from build123d import *

# Parameters (mm, degrees)
F0_W     = 250
F0_H     = 75
F1_DEPTH = 17.5
F3_DEPTH = 35.001
F4_R     = 9.5
F5_DEPTH = 50
F6_W     = 15
F6_H     = 150
F7_DEPTH = 37.501


with BuildPart() as f1:
    # F0 (on Right) → F1 (new body, symmetric)
    with BuildSketch(Plane.YZ):
        Rectangle(F0_W, F0_H)
    extrude(amount=F1_DEPTH, both=True)

    # F2 (on face) → F3 (cut, through all)
    with BuildSketch(Plane(origin=(-17.5, 0, 0), x_dir=(0, -1, 0), z_dir=(-1, 0, 0))):
        with BuildLine():
            ThreePointArc((-125, 37.5), (-59.748084, 27.923052), (0, 0))
            ThreePointArc((0, 0), (61.011045, -23.713184), (125, -37.5))
            Line((125, -37.5), (125, 37.5))
            Line((125, 37.5), (-125, 37.5))
        make_face()
        with BuildLine():
            Line((-125, -37.5), (76.611606, -37.5))
            ThreePointArc((76.611606, -37.5), (52.114015, -27.662953), (26.677744, -20.59927))
            ThreePointArc((26.677744, -20.59927), (-50.552427, -16.563242), (-125, -37.5))
        make_face()
        with BuildLine():
            ThreePointArc((26.677744, -20.59927), (-49.327107, -2.636934), (-125, -21.950044))
            Line((-125, -21.950044), (-125, -37.5))
            ThreePointArc((-125, -37.5), (-50.552427, -16.563242), (26.677744, -20.59927))
        make_face()
    extrude(amount=-F3_DEPTH, mode=Mode.SUBTRACT)

    # F4 (on face) → F5 (cut)
    with BuildSketch(Plane(origin=(0, 125, 0), x_dir=(-1, 0, 0), z_dir=(0, 1, 0))):
        with Locations((0, 17.31561)):
            Circle(F4_R)
    extrude(amount=-F5_DEPTH, mode=Mode.SUBTRACT)

    # F6 (on Top) → F7 (cut, through all)
    with BuildSketch(Plane.XY):
        with Locations((0.914634, -15.109161)):
            Rectangle(F6_W, F6_H)
    extrude(amount=-F7_DEPTH, mode=Mode.SUBTRACT)


solid = f1.part
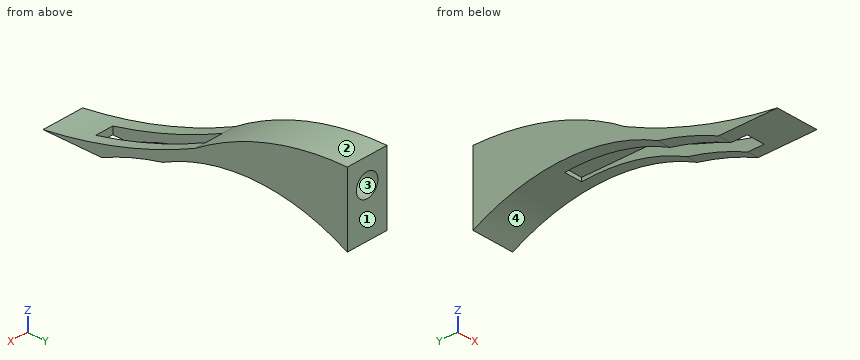
Read the model definition and answer for the solid it produces. Units are mm, in the model's axes. Face numbers are marked on the shaded views. Give positions to 0.01 mm unless a question says otherwise; leave off trailing zeros. Write each loop counter-clockwise with the first axis right and the second up, starting at its lowest first coordinate (ties: lowest second). Pieces come first, ordered by that corner, then holes. Notation, with made-up numbers: (-32, 41.5) -> (27, 41.5) arc R28 cw to (27, 61.5) -> close; hole circle Ø5 at (-10.75, 87.5). An arc over 180 degrees is marked (long way). Answer as a JSON object with one key per item and string values. Group by question number.
1) Find section B-B (z = -12.5). Write down the section's boundary in (x, y).
2) Find section D-D (y = -65). Write down the section's boundary in (x, z).
3) Find section A-A (x = 0). Write down the section's boundary in (y, z), and give its area (3 significant figures).
4) Each of these flat-tipped pins is pushed along its axis until it touches: P1, Ø1.9, axis at x = 0, z = -33.5, coming from the +Y side; P2, Ø1.5, axis at x = -4.5, y = -90, coming from the +Z side; P3, Ø10, axis at x = 9.5, y = -22, coming from the +Z side. Where does it stop, or does it pass through?
5) Consider L1, parallel to X at y = -56, z = -25; L2, parallel to Z at x = 0, y = 87.5; L3, parallel to Z at x = 0, y = 101. Determine where each line is inside the solid, lowest interval first. Write a range as from..to.
6) The mould has two halves that part along Y. Classify the marked faces 1, 2, 3 and 4: +Y half, -Y half, draft (parallel to the pull), parting line (faces both ways), or undercut.
7) Find section C-C (x = 14). Write down the section's boundary in (y, z), and give its area (3 significant figures).
Values follow:
{
 "1": {"outline": "(-17.5, -28.59) -> (-6.59, -28.59) -> (-6.59, -8.1) -> (-17.5, -8.1) -> close; (-17.5, 103.84) -> (17.5, 103.84) -> (17.5, 125) -> (-17.5, 125) -> close; (8.41, -28.59) -> (17.5, -28.59) -> (17.5, -8.1) -> (8.41, -8.1) -> close"},
 "2": {"outline": "(-17.5, -32.44) -> (-6.59, -32.44) -> (-6.59, -24.89) -> (-17.5, -24.89) -> close; (8.41, -32.44) -> (17.5, -32.44) -> (17.5, -24.89) -> (8.41, -24.89) -> close"},
 "3": {"outline": "(-125, -37.5) -> (-90.11, -37.5) -> (-90.11, -31.3) arc R413.44 cw to start; (0, 0) -> (59.89, 0) -> (59.89, -3.07) arc R163.62 cw to (125, -21.95) -> (125, 7.82) -> (75, 7.82) -> (75, 26.82) -> (125, 26.82) -> (125, 37.5) arc R227.08 ccw to start", "area": "2,980 mm2"},
 "4": {"P1": "stops at y = -90.11", "P2": "stops at z = -31.3", "P3": "stops at z = -7.74"},
 "5": {"L1": "x = -17.5..-6.59, 8.41..17.5", "L2": "z = -7.5..7.82, 26.82..34.38", "L3": "z = -11.5..7.82, 26.82..36.23"},
 "6": {"face 1": "+Y half", "face 2": "-Y half", "face 3": "draft", "face 4": "undercut"},
 "7": {"outline": "(-125, -37.5) -> (-76.61, -37.5) arc R238.02 cw to (-26.68, -20.6) arc R163.62 cw to (125, -21.95) -> (125, 37.5) arc R227.08 ccw to (0, 0) arc R413.44 cw to start", "area": "4,920 mm2"}
}
